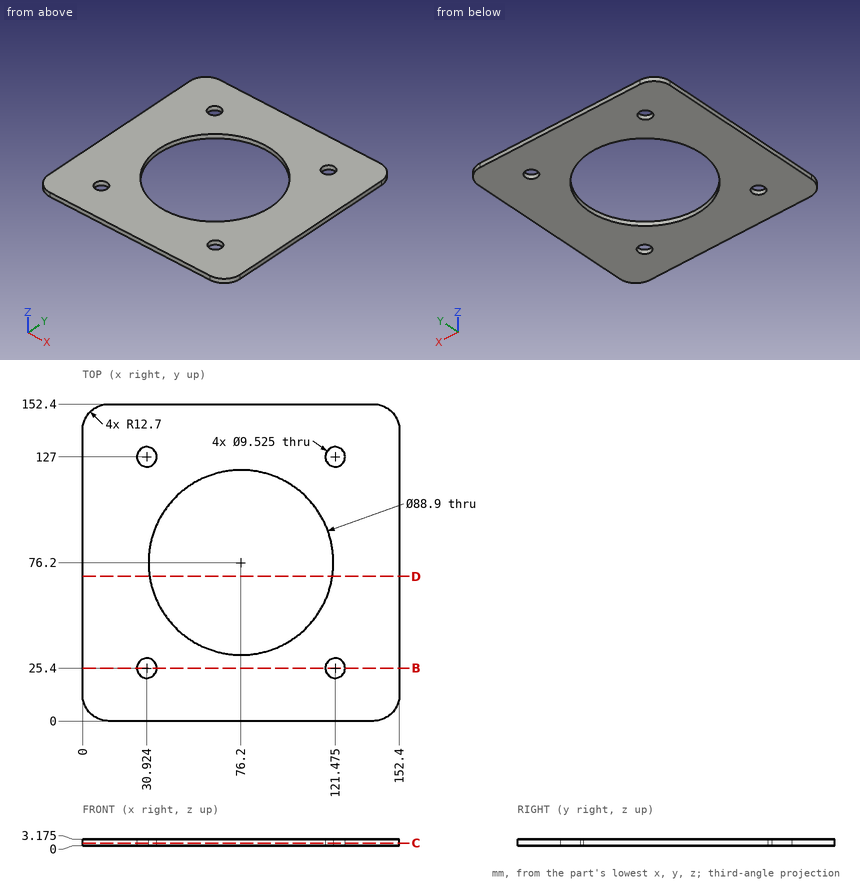
Geometry: see drawing. Coordinates: mm, zero at the bounding-box minimum. Coordinates: 2 decimals unless noted, no trailing zeros. Write each loop counter-clockwise with the first axis right and the second up, starting at its lowest first coordinate (ties: lowest second). Pieces come first, ordered by that corner, then holes.
1) Section B-B on y = 25.4. Output: boundary loops of the cut face in (x, z) (1 decimal).
2) Pin query (flat end, axial travel): pin 1 Ø11 at (x, y) = (30.92, 25.4) entering from -Z. Return the tip coordinate at first contact, or that it passes through.
3) Material intervals for line 1 along Y through (x, z) = (76.2, 2.1); line 2 along X through (y, z) = (58, 1.75) (1 decimal); line 3 along X through (y, z) = (21.5, 0.4) (1 decimal), sorted ascending.
4) Section C-C on z = 1.2. State how many separate pieces and enclosed holes the cut face has, and give its area (3 significant figures).
5) Section D-D on y = 69.5. Output: boundary loops of the cut face in (x, z) (1 decimal).
Check result:
1. outline: (0, 0) - (26.2, 0) - (26.2, 3.2) - (0, 3.2) - close; (35.7, 0) - (116.7, 0) - (116.7, 3.2) - (35.7, 3.2) - close; (126.2, 0) - (152.4, 0) - (152.4, 3.2) - (126.2, 3.2) - close
2. pin 1: stops at z = 0
3. line 1: y = 0 to 31.75, 120.65 to 152.4
3. line 2: x = 0 to 35.6, 116.8 to 152.4
3. line 3: x = 0 to 28.2, 33.7 to 118.7, 124.2 to 152.4
4. separate pieces: 1
4. enclosed holes: 5
4. area: 16,600 mm2
5. outline: (0, 0) - (32.3, 0) - (32.3, 3.2) - (0, 3.2) - close; (120.1, 0) - (152.4, 0) - (152.4, 3.2) - (120.1, 3.2) - close
